Input: part model. Units: mm. Frame: model coordinates. A direction names the side the tool comes from. Coordinates: 2 decimals unless noted, no trailing zeros. Order: outer loops, then holes, each group sorted by start corner. A loop starts at its lowest first (then second) coordinate and runs counter-clockwise, first axis right, second up. Notation, with made-up numbers: (-30.5, 32.25) -> (1.5, 32.25) arc R10 cw to (1.5, 43.25) -> close; hole circle Ø6 at (-19, -11). An arc over 180 degrees is marked (long way). Answer as CSV lines item,"result".
from build123d import *

# Parameters (mm, degrees)
BOSS_EXTRUDE1_DEPTH = 52.243773639
SKETCH2_W           = 26.940383964
SKETCH2_H           = 5.525205864
BOSS_EXTRUDE2_DEPTH = 2
FILLET1_R           = 5
FILLET3_R           = 1
FILLET4_R           = 5
SKETCH3_R           = 3.508090029
BOSS_EXTRUDE3_DEPTH = 2
FILLET5_R           = 5
FILLET6_R           = 5


# Some blends are built 0.0001 mm under size
with BuildPart() as part:
    # Sketch1 → Boss-Extrude1 (new body)
    with BuildSketch(Plane(origin=(0, 0, 0), x_dir=(1, 0, 0), z_dir=(0, 1, 0))):
        Polygon((13.470191982, 0), (-13.470191982, 0), (-13.470191982, 3), (-10, 3), (-10, 6), (-15, 6), (-15, 8), (15, 8), (15, 6), (10, 6), (10, 3), (13.470191982, 3), align=None)
    extrude(amount=BOSS_EXTRUDE1_DEPTH)

    # Sketch2 → Boss-Extrude2 (add)
    with BuildSketch(Plane.XZ):
        with Locations((0, -4.262602932)):
            Rectangle(SKETCH2_W, SKETCH2_H)
    extrude(amount=-BOSS_EXTRUDE2_DEPTH)

    # Fillet1
    fillet1_edges = [part.edges().sort_by_distance(p)[0] for p in [
        (10, 52.243773639, -4.5),
        (-10, 52.243773639, -4.5),
        (-15, 52.243773639, -7),
        (15, 52.243773639, -7),
    ]]
    fillet(fillet1_edges, radius=FILLET1_R - 0.0001)  # a hair under: the kernel refuses the full size

    # Fillet3
    fillet3_edges = [part.edges().sort_by_distance(p)[0] for p in [
        (13.470191982, 2, -4.5),
        (-13.470191982, 2, -4.5),
        (10, 2, -4.5),
        (-10, 2, -4.5),
    ]]
    fillet(fillet3_edges, radius=FILLET3_R)

    # Fillet4
    fillet4_edges = [part.edges().sort_by_distance(p)[0] for p in [
        (13.470191982, 52.243773639, -1.5),
        (-13.470191982, 52.243773639, -1.5),
    ]]
    fillet(fillet4_edges, radius=FILLET4_R)

    # Sketch3 → Boss-Extrude3 (add)
    with BuildSketch(Plane(origin=(0, 0, -8), x_dir=(-1, 0, 0), z_dir=(0, 0, -1))):
        with Locations(Location((0, 32, 0), (0, 0, 180))):
            Circle(SKETCH3_R)
    extrude(amount=BOSS_EXTRUDE3_DEPTH)

    # Fillet5
    # the kernel refuses this fillet: 5 mm, written as the material it adds along each edge
    with BuildSketch(Plane(origin=(0, 32, -8), x_dir=(1, 0, 0), z_dir=(0, 1, 0))) as fillet5_piece_1:
        with BuildLine():
            CenterArc((7.508090029, 5), FILLET5_R, 216.869897646, 53.130102354)
            Line((3.508090029, 2), (3.428090029, 1.94))
            ThreePointArc((3.428090029, 1.94), (3.408090029, 1), (3.408090029, 0))
            Line((3.408090029, 0), (3.508090029, -0.1))
            Line((3.508090029, -0.1), (7.508090029, -0.1))
            Line((7.508090029, -0.1), (7.508090029, 0))
        make_face()
    revolve(axis=Axis((0, 32, -8), (0, 0, -1)))

    # Fillet6
    fillet6_edges = [part.edges().sort_by_distance(p)[0] for p in [
        (-3.508090029, 32, -10),
    ]]
    fillet(fillet6_edges, radius=FILLET6_R)


solid = part.part
1. Cut plane C-C (x = -11.5). Return the cut outline in (y, z).
Findings:
outline,"(0, -8) -> (52.01, -8) -> (52.01, -6) -> (2, -6) -> (2, -3) -> (51.22, -3) -> (51.22, 0) -> (0, 0) -> close"
2. Cut plane B-B (z = -5.25). Return the cut outline in (x, y).
Findings:
outline,"(-13.47, 0) -> (13.47, 0) -> (13.47, 1) arc R1 ccw to (12.47, 2) -> (11, 2) arc R1 cw to (10, 3) -> (10, 47.24) arc R5 ccw to (5, 52.24) -> (-5, 52.24) arc R5 ccw to (-10, 47.24) -> (-10, 3) arc R1 cw to (-11, 2) -> (-12.47, 2) arc R1 ccw to (-13.47, 1) -> close"
3. Contact query for flat-ended pins moving along their axis: pin 1 (4 mm diameter, centred on x = -10, y = 34, fed in from -Z); pin 2 (3 mm diameter, centred on x = 4, y = 31.5, fed in from -Z); pin 3 (1.2 mm diameter, centred on x = -12, z = -4, fed in from +Y). Output: stop coordinate, or through.
Findings:
pin 1,"stops at z = -8"
pin 2,"stops at z = -9.89"
pin 3,"stops at y = 2"
4. Mould query, pull axis Z, two halves, no side actions, for faces 1 (the face through (0, 20, -8)), 2 (the face through (-10.285, 2.301, -4.479)), 3 (the face through (12.044, 50.74, -1.479)). Classes: released by +Z, released by -Z, zero draft, split by the parting line, or undercut.
Findings:
face 1,"released by -Z"
face 2,"undercut"
face 3,"zero draft"
5. Ray query, line 1 along Z through (x, y) = (-4.5, 39); line 2 along Z through (x, y) = (12.25, 42.5); line 3 along X through (y, z) = (27, -1.5). Return the intervals inside material, ascending.
Findings:
line 1,"z = -8 to 0"
line 2,"z = -8 to -6, -3 to 0"
line 3,"x = -13.47 to 13.47"
6. Cut plane A-A (y = 5). Return the cut outline in (x, z), plus the area to 3 significant figures.
Findings:
outline,"(-15, -8) -> (15, -8) -> (15, -6) -> (10, -6) -> (10, -3) -> (13.47, -3) -> (13.47, 0) -> (-13.47, 0) -> (-13.47, -3) -> (-10, -3) -> (-10, -6) -> (-15, -6) -> close"
area,"201 mm2"
7. Reachability of faces 4 (the face through (13.47, 23, -1)), 5 (the face through (-8.574, 50.74, -4.521)), 6 (the face through (0, 0, -4)), 7 (the face through (10, 25, -5)), 8 (the face through (-13.47, 23, -2)) from +Z, -Z, +X, -X, +Y, -Y: full face, straight path, thin tool, end or side. Return the list, or none.
Findings:
face 4,"+Z, +X, +Y, -Y"
face 5,"-X, +Y"
face 6,"+Z, -Z, +X, -X, -Y"
face 7,"+X, +Y"
face 8,"+Z, -X, +Y, -Y"
